Verification items for the finished model (mm, model axes). Round coordinates to 2 decimals unless told otherwise and drop trailing zeros. Order: outer loops, then holes, each group sorted by start corner. A loop starts at its lowest first (then second) coordinate and runs counter-clockwise, first axis right, second up. Notation, with made-up numbers: (57, -33.5) -> (107, -33.5) arc R19 ccw to (107, -24.5) -> close; hole circle Ø5 at (-9, -36). An arc over 180 degrees is marked (long way). Return JSON: item names as keys, results as strings. Group by question number.
Item 1: Depth check by flat-ended pin: pin 1 Ø7.5 at (y, z) = (57, 17.5) entering from -X; pin 2 Ø7.5 at (x, z) = (214.5, 18) entering from -Y; pin 3 Ø10 at (y, z) = (-365.5, 16) entering from +X. Enter the tip coordinate at first touch or a pass-through.
Item 2: Scan lines: probe 1 along X at (y, z) = (-434, 21.75); probe 2 along X at (y, z) = (-12, 8); probe 3 along X at (y, z) = (143, 3.25). Record each from-to range of solid material in increasing order. Write a range as from..to.
Item 3: Sectioned sample at B-B on y = -168. Record the cut outline in (x, z), plus the area to 3 significant figures.
Item 4: Sectioned sample at C-C on z = 4.5. Give the number of separate pieces and of enclosed holes in the cut face, plus the area to 3 significant figures.
Item 5: Sectioned sample at A-A on x = -120. Record the cut outline in (y, z).
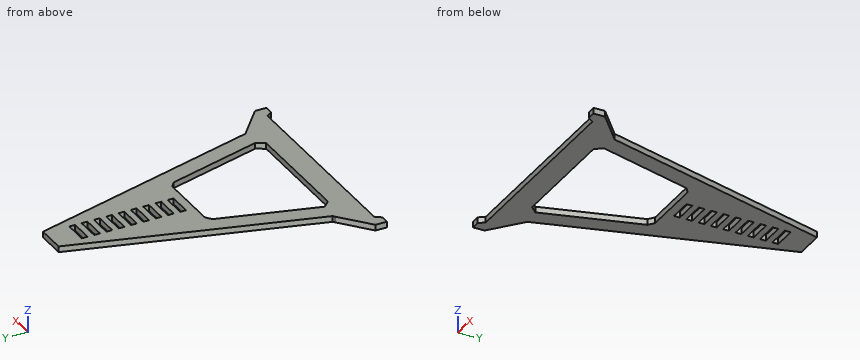
```python
from build123d import *
from OCP.BRepFilletAPI import BRepFilletAPI_MakeChamfer

# Parameters (mm, degrees)
BOSS_EXTRUDE1_DEPTH = 25.4
CHAMFER1_SIZE       = 38.1
CHAMFER1_SIZE2      = 30.889863159
CHAMFER2_SIZE       = 20.32
CHAMFER2_SIZE2      = 19.275364183
SKETCH2_W           = 101.6
SKETCH2_H           = 25.4
CUT_EXTRUDE2_DEPTH  = 775.10421823
LPATTERN1_COUNT     = 2
LPATTERN1_PITCH     = 106.68


with BuildPart() as part:
    # Sketch1 → Boss-Extrude1 (new body)
    with BuildSketch(Plane.XY):
        Polygon((0, 597.4769356), (0, 0), (152.4, 0), (285.215433829, -472.186), (0, -472.186), (0, -573.786), (415.976251613, -573.786), (433.57458701, -573.786), (452.189239648, -599.186), (469.838640091, -599.186), (489.457166752, -599.186), (489.457166752, -548.960321271), (361.710639116, -441.768257047), (353.995711594, -435.294664209), (63.5, 597.4769356), align=None)
    boss_extrude1 = extrude(amount=BOSS_EXTRUDE1_DEPTH)

    # Mirror1: Boss-Extrude1 across plane
    add(boss_extrude1.mirror(Plane(origin=(0, 0, 25.4), x_dir=(0, 0, 1), z_dir=(1, 0, 0))))

    # Chamfer1: one chamfer whose edges measure the first distance from different faces: ONE call of the kernel's chamfer builder (chamfer() names one face for all edges)
    chamfer1_edges_1 = [part.edges().sort_by_distance(p)[0] for p in [
        (285.215433829, -472.186, 12.7),
    ]]
    chamfer1_side_1 = [part.faces().sort_by_distance(p)[0] for p in [
        (218.807716914, -236.093, 12.7),
    ]]
    chamfer1_edges_2 = [part.edges().sort_by_distance(p)[0] for p in [
        (-285.215433829, -472.186, 12.7),
    ]]
    chamfer1_side_2 = [part.faces().sort_by_distance(p)[0] for p in [
        (0, -472.186, 12.7),
    ]]
    chamfer1 = BRepFilletAPI_MakeChamfer(part.part.solid().wrapped)
    for e in chamfer1_edges_1:
        chamfer1.Add(CHAMFER1_SIZE, CHAMFER1_SIZE2, e.wrapped, chamfer1_side_1[0].wrapped)  # the first distance lies on this face
    for e in chamfer1_edges_2:
        chamfer1.Add(CHAMFER1_SIZE, CHAMFER1_SIZE2, e.wrapped, chamfer1_side_2[0].wrapped)  # the first distance lies on this face
    add(Compound.cast(chamfer1.Shape()), mode=Mode.REPLACE)

    # Chamfer2: one chamfer whose edges measure the first distance from different faces: ONE call of the kernel's chamfer builder (chamfer() names one face for all edges)
    chamfer2_edges_1 = [part.edges().sort_by_distance(p)[0] for p in [
        (152.4, 0, 12.7),
    ]]
    chamfer2_side_1 = [part.faces().sort_by_distance(p)[0] for p in [
        (0, 0, 12.7),
    ]]
    chamfer2_edges_2 = [part.edges().sort_by_distance(p)[0] for p in [
        (-152.4, 0, 12.7),
    ]]
    chamfer2_side_2 = [part.faces().sort_by_distance(p)[0] for p in [
        (-214.625687132, -221.225029782, 12.7),
    ]]
    chamfer2 = BRepFilletAPI_MakeChamfer(part.part.solid().wrapped)
    for e in chamfer2_edges_1:
        chamfer2.Add(CHAMFER2_SIZE, CHAMFER2_SIZE2, e.wrapped, chamfer2_side_1[0].wrapped)  # the first distance lies on this face
    for e in chamfer2_edges_2:
        chamfer2.Add(CHAMFER2_SIZE, CHAMFER2_SIZE2, e.wrapped, chamfer2_side_2[0].wrapped)  # the first distance lies on this face
    add(Compound.cast(chamfer2.Shape()), mode=Mode.REPLACE)

    # Sketch2 → Cut-Extrude2 (cut, through all)
    with BuildSketch(Plane.XY.offset(25.4)):
        with Locations((0, 50.8)):
            Rectangle(SKETCH2_W, SKETCH2_H)
        with Locations((0, 104.14)):
            Rectangle(SKETCH2_W, SKETCH2_H)
        with Locations((0, 157.48)):
            Rectangle(SKETCH2_W, SKETCH2_H)
        with Locations((0, 210.82)):
            Rectangle(SKETCH2_W, SKETCH2_H)
        with Locations((0, 264.16)):
            Rectangle(SKETCH2_W, SKETCH2_H)
        with Locations((0, 317.5)):
            Rectangle(SKETCH2_W, SKETCH2_H)
        with Locations((0, 370.84)):
            Rectangle(SKETCH2_W, SKETCH2_H)
    cut_extrude2 = extrude(amount=-CUT_EXTRUDE2_DEPTH, mode=Mode.SUBTRACT)

    # LPattern1: Cut-Extrude2 ×2
    with Locations(*[(0, i * LPATTERN1_PITCH, 0) for i in range(1, LPATTERN1_COUNT)]):
        add(cut_extrude2, mode=Mode.SUBTRACT)


solid = part.part
```
Recorded:
{
 "1": {"pin 1": "x = -216.58", "pin 2": "y = -573.79", "pin 3": "x = 335.77"},
 "2": {"probe 1": "-353.63..-274.47, 274.47..353.63", "probe 2": "-234.93..-148.32, 148.6..234.93", "probe 3": "-191.33..191.33"},
 "3": {"outline": "(-278.81, 0) -> (-199.65, 0) -> (-199.65, 25.4) -> (-278.81, 25.4) -> close; (199.65, 0) -> (278.81, 0) -> (278.81, 25.4) -> (199.65, 25.4) -> close", "area": "4,020 mm²"},
 "4": {"separate pieces": "1", "enclosed holes": "10", "area": "325,000 mm²"},
 "5": {"outline": "(-573.79, 0) -> (-472.19, 0) -> (-472.19, 25.4) -> (-573.79, 25.4) -> close; (0, 0) -> (396.61, 0) -> (396.61, 25.4) -> (0, 25.4) -> close"}
}
